from build123d import *

# Parameters (mm, degrees)
BOSS_EXTRUDE1_DEPTH      = 23
BOSS_EXTRUDE2_DEPTH      = 2
BOSS_EXTRUDE3_DEPTH      = 15
BOSS_EXTRUDE3_DEPTH_BACK = 70


with BuildPart() as part:
    # Sketch1 → Boss-Extrude1 (new body)
    with BuildSketch(Plane.XY):
        Polygon((38, 50), (40, 45), (75, 45), (75, 5), (40, 5), (38, 0), (0, 0), (0, 50), align=None)
    extrude(amount=BOSS_EXTRUDE1_DEPTH)

    # Sketch2 → Boss-Extrude2 (add)
    with BuildSketch(Plane(origin=(0, 0, 0), x_dir=(-1, 0, 0), z_dir=(0, 0, -1))):
        with BuildLine():
            Line((-24.376413311, 54.915521171), (-27.283060583, 50))
            Line((-27.283060583, 50), (-23.283060583, 50))
            Line((-23.283060583, 50), (-23.283060583, 55.116465729))
            add(Edge.make_bspline(
                [(-23.283060583, 55.116465729), (-22.783060583, 55.344163988), (-21.783060583, 55.799560505), (-20.783060583, 55.344163988), (-20.283060583, 55.116465729)],
                knots=[0, 0, 0, 0, 0.5, 1, 1, 1, 1], degree=3))
            Line((-20.283060583, 55.116465729), (-20.283060583, 50))
            Line((-20.283060583, 50), (-16.283060583, 50))
            Line((-16.283060583, 50), (-19.189707855, 54.915521171))
            add(Edge.make_bspline(
                [(-19.189707855, 54.915521171), (-19.646594621, 55.426566158), (-20.482340041, 56.318719988), (-20.795963928, 56.329848385), (-21.430200541, 56.439930134), (-21.783060583, 56.416877275)],
                knots=[0, 0, 0, 0, 0.318153244, 0.553620623, 0.81642651, 0.81642651, 0.81642651, 0.81642651], degree=3))
            add(Edge.make_bspline(
                [(-24.376413311, 54.915521171), (-23.919526545, 55.426566158), (-23.083781124, 56.318719988), (-22.770157237, 56.329848385), (-22.135920624, 56.439930134), (-21.783060583, 56.416877275)],
                knots=[0, 0, 0, 0, 0.318153244, 0.553620623, 0.81642651, 0.81642651, 0.81642651, 0.81642651], degree=3))
        make_face()
    boss_extrude2 = extrude(amount=-BOSS_EXTRUDE2_DEPTH)

    # Mirror1: Boss-Extrude2 across plane
    add(boss_extrude2.mirror(Plane.ZX.offset(25)))

    # Sketch3 → Boss-Extrude3 (add, two sides: drawn at the far end of the back side and taken through both)
    with BuildSketch(Plane.XZ.offset(-BOSS_EXTRUDE3_DEPTH_BACK)):
        Polygon((5.3022214, 11.32), (4.55166605, 12.62), (3.05055535, 12.62), (2.3, 11.32), (3.05055535, 10.02), (4.55166605, 10.02), align=None)
    extrude(amount=BOSS_EXTRUDE3_DEPTH + BOSS_EXTRUDE3_DEPTH_BACK)


solid = part.part
Geometry check sheet. Reference: the model listing, model coordinates, mm. A direction names the side the tool comes from. Give positions to 0.01 mm unless a question says otherwise; leave off trailing zeros. Order: outer loops, then holes, each group sorted by start corner. A loop starts at its lowest first (then second) coordinate and runs counter-clockwise, first axis right, second up.
1) Cross-section at D-D (x = 47). Record the boundary of the cut face in (y, z).
Results are:
outline: (5, 0) - (45, 0) - (45, 23) - (5, 23) - close
2) Cross-section at B-B (y = -2). Record the boundary of the cut face in (x, z).
Results are:
outline: (2.3, 11.32) - (3.05, 10.02) - (4.55, 10.02) - (5.3, 11.32) - (4.55, 12.62) - (3.05, 12.62) - close; (17.47, 0) - (20.28, 0) - (20.28, 2) - (17.47, 2) - close; (23.28, 0) - (26.1, 0) - (26.1, 2) - (23.28, 2) - close
3) Gauge pin test, flat ends, axial feed: pin 1 (2 mm diameter, centred on x = 55.5, z = 14, fed in from -Y); pin 2 (8 mm diameter, centred on x = 43.5, z = 10.5, fed in from +Y); pin 3 (2 mm diameter, centred on y = 51.5, z = 1, fed in from -X); pin 4 (5 mm diameter, centred on x = 20.5, y = -2, fed in from +Z). Record the tip position at first contact, or that the pin passes through.
Results are:
pin 1: stops at y = 5
pin 2: stops at y = 46.25
pin 3: stops at x = 16.58
pin 4: stops at z = 23
4) Draft check along Y on faces 1 (the flat face through (0, 25, 11)), 2 (the flat face through (17.7, 52.4, 1)), 3 (the flat face through (20.283, -3, 1)). Enter one of: released by +Y, released by -Y, zero draft, split by the parting line, or undercut.
Results are:
face 1: zero draft
face 2: released by +Y
face 3: undercut
5) Tool access check on faces 4 (the flat face through (19, 53, 2)), 5 (the flat face through (58, 5, 11)), 6 (the flat face through (57, 45, 11)), 7 (the flat face through (75, 25, 11)), 8 (the flat face through (20.283, 53, 1)). Record the directions out of +Z, -Z, +X, -X, +Y, -Y that give a thin tool (end or side, any length) a straight path to the whole face; none if there is none.
Results are:
face 4: +Z, +X, -X, +Y
face 5: +Z, -Z, +X, -Y
face 6: +Z, -Z, +X, +Y
face 7: +Z, -Z, +X, +Y, -Y
face 8: +Z, -Z
6) Cross-section at C-C (x = 10.5). Record the boundary of the cut face in (y, z).
Results are:
outline: (0, 0) - (50, 0) - (50, 23) - (0, 23) - close
7) Material ranges on probe 1 along Y at (x, z) = (13, 10.25); probe 2 along Y at (x, z) = (55, 17); probe 3 along X at (y, z) = (47.5, 6.75), recorded low to high.
Results are:
probe 1: y = 0 to 50
probe 2: y = 5 to 45
probe 3: x = 0 to 39
8) Cross-section at A-A (z = 6.5). Record the boundary of the cut face in (x, y), then the cut area to 3 significant figures.
Results are:
outline: (0, 0) - (38, 0) - (40, 5) - (75, 5) - (75, 45) - (40, 45) - (38, 50) - (0, 50) - close
area: 3,390 mm2
